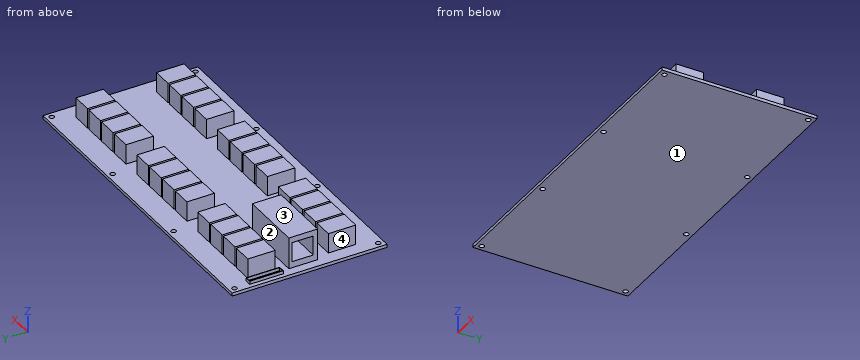
from build123d import *

# Parameters (mm, degrees)
SKETCH1_W                       = 262.255
SKETCH1_H                       = 124.333
BOSS_EXTRUDE1_DEPTH             = 2.54
F_5_32_0_15625_DIAMETER_HOLE1_D = 3.96875
SKETCH12_W                      = 5.08
SKETCH12_H                      = 26.924
SKETCH12_W_2                    = 4.367686067
SKETCH12_H_2                    = 26.272785271
BOSS_EXTRUDE2_DEPTH             = 2.54
SKETCH13_W                      = 50.710492808
SKETCH13_H                      = 23.078831344
BOSS_EXTRUDE3_DEPTH             = 25.4
SKETCH14_W                      = 15.728561486
SKETCH14_H                      = 17.117120152
CUT_EXTRUDE1_DEPTH              = 25.4
SKETCH16_W                      = 16.002
SKETCH16_H                      = 21.9964
BOSS_EXTRUDE5_DEPTH             = 16.002
LPATTERN1_COUNT                 = 4
LPATTERN1_PITCH                 = 17.78
MIRROR1_COPY_1_SKETCH_W         = 16.002
MIRROR1_COPY_1_SKETCH_H         = 21.9964
MIRROR1_COPY_1_DEPTH            = 16.002
MIRROR1_COPY_2_SKETCH_W         = 16.002
MIRROR1_COPY_2_SKETCH_H         = 21.9964
MIRROR1_COPY_2_DEPTH            = 16.002
MIRROR1_COPY_3_SKETCH_W         = 16.002
MIRROR1_COPY_3_SKETCH_H         = 21.9964
MIRROR1_COPY_3_DEPTH            = 16.002


with BuildPart() as part:
    # Sketch1 → Boss-Extrude1 (new body)
    with BuildSketch(Plane.XY):
        with Locations((131.1275, 62.1665)):
            Rectangle(SKETCH1_W, SKETCH1_H)
    extrude(amount=BOSS_EXTRUDE1_DEPTH)

    # 5/32 (0.15625) Diameter Hole1 (through all)
    with Locations(Plane.XY.offset(2.54)):
        with Locations((4.445, 119.888), (88.9, 119.888), (173.355, 119.888), (257.81, 119.888), (4.445, 4.445), (88.9, 4.445), (173.355, 4.445), (257.81, 4.445)):
            Hole(F_5_32_0_15625_DIAMETER_HOLE1_D / 2)

    # Sketch12 → Boss-Extrude2 (add)
    with BuildSketch(Plane.XY.offset(2.54)):
        with Locations((6.044810111, 94.689164449)):
            Rectangle(SKETCH12_W, SKETCH12_H)
        with Locations((6.063998692, 94.748985924)):
            Rectangle(SKETCH12_W_2, SKETCH12_H_2, mode=Mode.SUBTRACT)
    extrude(amount=BOSS_EXTRUDE2_DEPTH)

    # Sketch13 → Boss-Extrude3 (add)
    with BuildSketch(Plane.XY.offset(2.54)):
        with Locations((32.501526889, 63.129188548)):
            Rectangle(SKETCH13_W, SKETCH13_H)
    extrude(amount=BOSS_EXTRUDE3_DEPTH)

    # Sketch14 → Cut-Extrude1 (cut)
    with BuildSketch(Plane.ZY.offset(-7.146280485)):
        with Locations((15.411737976, 63.690176449)):
            Rectangle(SKETCH14_W, SKETCH14_H)
    extrude(amount=-CUT_EXTRUDE1_DEPTH, mode=Mode.SUBTRACT)

    # Sketch16 → Boss-Extrude5 (add)
    with BuildSketch(Plane.XY.offset(2.54)):
        with Locations((103.251, 94.491464858)):
            Rectangle(SKETCH16_W, SKETCH16_H)
        with Locations((18.796, 94.491464858)):
            Rectangle(SKETCH16_W, SKETCH16_H)
        with Locations((187.706, 94.491464858)):
            Rectangle(SKETCH16_W, SKETCH16_H)
    boss_extrude5 = extrude(amount=BOSS_EXTRUDE5_DEPTH)

    # LPattern1: Boss-Extrude5 ×4
    with Locations(*[(i * LPATTERN1_PITCH, 0, 0) for i in range(1, LPATTERN1_COUNT)]):
        add(boss_extrude5)

    # Mirror1: Boss-Extrude5 across plane
    add(boss_extrude5.mirror(Plane.ZX.offset(62.1665)))

    # Mirror1 copy 1 sketch → Mirror1 copy 1 (add)
    with BuildSketch(Plane(origin=(17.78, 124.333, 2.54), x_dir=(1, 0, 0), z_dir=(0, 0, 1))):
        with Locations((103.251, -94.491464858)):
            Rectangle(MIRROR1_COPY_1_SKETCH_W, MIRROR1_COPY_1_SKETCH_H)
        with Locations((18.796, -94.491464858)):
            Rectangle(MIRROR1_COPY_1_SKETCH_W, MIRROR1_COPY_1_SKETCH_H)
        with Locations((187.706, -94.491464858)):
            Rectangle(MIRROR1_COPY_1_SKETCH_W, MIRROR1_COPY_1_SKETCH_H)
    extrude(amount=MIRROR1_COPY_1_DEPTH)

    # Mirror1 copy 2 sketch → Mirror1 copy 2 (add)
    with BuildSketch(Plane(origin=(35.56, 124.333, 2.54), x_dir=(1, 0, 0), z_dir=(0, 0, 1))):
        with Locations((103.251, -94.491464858)):
            Rectangle(MIRROR1_COPY_2_SKETCH_W, MIRROR1_COPY_2_SKETCH_H)
        with Locations((18.796, -94.491464858)):
            Rectangle(MIRROR1_COPY_2_SKETCH_W, MIRROR1_COPY_2_SKETCH_H)
        with Locations((187.706, -94.491464858)):
            Rectangle(MIRROR1_COPY_2_SKETCH_W, MIRROR1_COPY_2_SKETCH_H)
    extrude(amount=MIRROR1_COPY_2_DEPTH)

    # Mirror1 copy 3 sketch → Mirror1 copy 3 (add)
    with BuildSketch(Plane(origin=(53.34, 124.333, 2.54), x_dir=(1, 0, 0), z_dir=(0, 0, 1))):
        with Locations((103.251, -94.491464858)):
            Rectangle(MIRROR1_COPY_3_SKETCH_W, MIRROR1_COPY_3_SKETCH_H)
        with Locations((18.796, -94.491464858)):
            Rectangle(MIRROR1_COPY_3_SKETCH_W, MIRROR1_COPY_3_SKETCH_H)
        with Locations((187.706, -94.491464858)):
            Rectangle(MIRROR1_COPY_3_SKETCH_W, MIRROR1_COPY_3_SKETCH_H)
    extrude(amount=MIRROR1_COPY_3_DEPTH)


solid = part.part
Can you work these out from the model? Positions are in its coordinate system, mm. Face numbers are marked on the shaded views. A direction names the side the tool comes from. Round coordinates to 2 decimals unless told otherwise and drop trailing zeros. Write each loop counter-clockwise with the first axis right and the second up, starting at its lowest first coordinate (ties: lowest second). Pieces come first, ordered by that corner, then holes. Notation, with made-up numbers: (89, -38) -> (134, -38) arc R19 cw to (134, -32) -> close; hole circle Ø8 at (77.5, -7). An arc over 180 degrees is marked (long way). One line per question, with ' | ' between items. Start each with the question number.
1) I'm going to push flat-ended pins straight in: P1, Ø8, axis at x = 225.5, z = 12.5, coming from the -Y side; P2, Ø4.5, axis at x = 257.81, y = 119.888, coming from the -Z side; P3, Ø1, axis at y = 34, z = 16.5, coming from the +X side; P4, Ø13, axis at x = 37, y = 35.5, coming from the +Z side. Where does each tip first touch, or does it pass through?
2) On a 3-axis mill with a long thin cutter (end or side, diameter ignored), from which of +Z, -Z, +X, -X, +Y, -Y can I reach the whole of each face in a straight line? I mean the marked faces 3 and 4. Say none if no direction works.
3) Suppose I cut it at C-C on x = 122. Write out the boundary of the cut face in (y, z).
4) Suppose I cut it at B-B on z = 13. Count the separate pieces of the cut face and the enclosed holes in it, then the cut area to 3 significant figures.
5) I need wall thicknesses on line 1 (Y direction, x = 257.81, z = 1.3); line 2 (Y direction, x = 219.5, z = 4.25); line 3 (Z direction, x = 80.5, y = 116.5). Which ranges of each line are inside material? Lowest first, please. Write a range as [from, to].
6) If we mould it in two halves opening along Y, with no side actions, what happens to the marked faces 1 and 2? For each: released by +Y, released by -Y, zero draft, split by the parting line, or undercut.
7) Suppose I cut it at A-A on y = 60.5. Write out the boundary of the cut face in (x, z) (3 decimals), then the cut area to 3 significant figures.
Return value:
1) P1: stops at y = 18.84 | P2: stops at z = 0 | P3: stops at x = 249.05 | P4: stops at z = 18.54
2) face 3: +Z, +X, -X, +Y, -Y | face 4: +Z, -X, -Y
3) outline: (0, 0) -> (124.33, 0) -> (124.33, 2.54) -> (105.49, 2.54) -> (105.49, 18.54) -> (83.49, 18.54) -> (83.49, 2.54) -> (40.84, 2.54) -> (40.84, 18.54) -> (18.84, 18.54) -> (18.84, 2.54) -> (0, 2.54) -> close
4) separate pieces: 25 | enclosed holes: 0 | area: 9,180 mm2
5) line 1: y = [0, 2.46], [6.43, 117.9], [121.87, 124.33] | line 2: y = [18.84, 40.84], [83.49, 105.49] | line 3: z = [0, 2.54]
6) face 1: zero draft | face 2: undercut
7) outline: (0, 0) -> (262.255, 0) -> (262.255, 2.54) -> (57.857, 2.54) -> (57.857, 27.94) -> (7.146, 27.94) -> (7.146, 23.276) -> (32.546, 23.276) -> (32.546, 7.547) -> (7.146, 7.547) -> (7.146, 2.54) -> (0, 2.54) -> close | area: 1,550 mm2
